Could you check a few things on this model? Use its own coordinates, in mm. A direction names the side the tool comes from. Round coordinates to 2 decimals unless told otherwise and drop trailing zeros. Loops run counter-clockwise (first coordinate to the right, second up) from the corner with the lowest first, then second, coordinate; pieces in that order, holes last. Notation, with made-up numbers: M 27,50.25 L 60,50.25 A23 ccw 60,63.25 Z; hole C 6.25,21 d11. An arc over 180 degrees is marked long. Answer in a Markdown table with one row per item.
```python
from build123d import *

# Parameters (mm, degrees)
EXTRUDE_1_DEPTH = 5


with BuildPart() as part:
    # 草图1 → 凸台-拉伸1 (new body)
    with BuildSketch(Plane(origin=(0, 0, 0), x_dir=(1, 0, 0), z_dir=(0, 1, 0))):
        Polygon((35, 290), (40, 290), (40, 230), (35, 230), (35, 180), (40, 180), (40, 110), (35, 110), (35, 60), (40, 60), (40, 0), (35, 0), (35, -5), (5, -5), (5, 0), (0, 0), (0, 60), (5, 60), (5, 110), (0, 110), (0, 180), (5, 180), (5, 230), (0, 230), (0, 290), (5, 290), (5, 295), (35, 295), align=None)
    extrude(amount=EXTRUDE_1_DEPTH)


solid = part.part
```
1) I need wall thicknesses on line 1 (Z direction, x = 35.5, y = 1.1); line 2 (X direction, y = 2.65, z = -103). Which ranges of each line are inside material? Lowest first, please.
Computed:
| item | result |
|---|---|
| line 1 | z = -290 to -230, -180 to -110, -60 to 0 |
| line 2 | x = 5 to 35 |
2) I want a section at A-A, the plane y = 2.45. Please give me the cut outline in (x, z).
Computed:
| item | result |
|---|---|
| outline | M 0,-290 L 5,-290 L 5,-295 L 35,-295 L 35,-290 L 40,-290 L 40,-230 L 35,-230 L 35,-180 L 40,-180 L 40,-110 L 35,-110 L 35,-60 L 40,-60 L 40,0 L 35,0 L 35,5 L 5,5 L 5,0 L 0,0 L 0,-60 L 5,-60 L 5,-110 L 0,-110 L 0,-180 L 5,-180 L 5,-230 L 0,-230 Z |
3) I want a section at B-B, the plane z = -74.5. Please give me the cut outline in (x, y), plus the area to 3 significant figures.
Computed:
| item | result |
|---|---|
| outline | M 5,0 L 35,0 L 35,5 L 5,5 Z |
| area | 150 mm² |
4) If we mould it in two halves opening along Z, with no side actions, what happens to faces 4 (the face through (2, 2, -290)), 5 (the face through (0, 2, -145)), 6 (the face through (35, 2, -205))? For each: released by +Z, released by -Z, zero draft, split by the parting line, or undercut.
Computed:
| item | result |
|---|---|
| face 4 | released by -Z |
| face 5 | zero draft |
| face 6 | undercut |
5) Which directions (+Z, -Z, +X, -X, +Y, -Y) give clear straight access to the entire face, cutting with the end or side of a thin tool? Please do faces 1 (the face through (3, 2, -230)), 2 (the face through (37, 2, -290)), 3 (the face through (3, 2, 0)).
Computed:
| item | result |
|---|---|
| face 1 | -X, +Y, -Y |
| face 2 | -Z, +X, +Y, -Y |
| face 3 | +Z, -X, +Y, -Y |
6) Will these pins go through, and if not, where does the flat tip stop? P1, Ø5, axis at x = 24, z = -37, coming from the -Y side; P2, Ø1.5, axis at y = 1.5, z = -77, coming from the -X side; P3, Ø1.5, axis at y = 3, z = -202.5, coming from the +X side; P4, Ø2.5, axis at x = 37, y = 3.5, coming from the -Z side.
Computed:
| item | result |
|---|---|
| P1 | stops at y = 0 |
| P2 | stops at x = 5 |
| P3 | stops at x = 35 |
| P4 | stops at z = -290 |
